```python
from build123d import *

# Parameters (mm, degrees)
SKETCH1_W                      = 155
SKETCH1_H                      = 290
BASE_FLANGE1_DEPTH             = 5
EDGE_FLANGE1_STRIP_W           = 36
EDGE_FLANGE1_STRIP_H           = 5
EDGE_FLANGE1_STRIP_CUT_DEPTH   = 290
EDGE_FLANGE1_STRIP_2_W         = 36
EDGE_FLANGE1_STRIP_2_H         = 5
EDGE_FLANGE1_STRIP_CUT_2_DEPTH = 290
EDGE_FLANGE1_DEPTH             = 290
EDGE_FLANGE1_BEND_DEPTH        = 290


# Sheet-metal steps are written as plain solids
with BuildPart() as part:
    # Sketch1 → Base-Flange1 (new body)
    with BuildSketch(Plane(origin=(0, 0, 0), x_dir=(1, 0, 0), z_dir=(0, 1, 0))):
        Rectangle(SKETCH1_W, SKETCH1_H)
    extrude(amount=-BASE_FLANGE1_DEPTH)

    # Edge-Flange1 strip (across the edge) → Edge-Flange1 strip cut (cut)
    with BuildSketch(Plane(origin=(77.5, -5, -145), x_dir=(-1, 0, 0), z_dir=(0, 0, 1))):
        with Locations((-5, -2.5)):
            Rectangle(EDGE_FLANGE1_STRIP_W, EDGE_FLANGE1_STRIP_H)
    extrude(amount=EDGE_FLANGE1_STRIP_CUT_DEPTH, mode=Mode.SUBTRACT)

    # Edge-Flange1 strip 2 (across the edge) → Edge-Flange1 strip cut 2 (cut)
    with BuildSketch(Plane(origin=(-77.5, -5, 145), x_dir=(1, 0, 0), z_dir=(0, 0, -1))):
        with Locations((-5, -2.5)):
            Rectangle(EDGE_FLANGE1_STRIP_2_W, EDGE_FLANGE1_STRIP_2_H)
    extrude(amount=EDGE_FLANGE1_STRIP_CUT_2_DEPTH, mode=Mode.SUBTRACT)

    # Edge-Flange1 section (across the edge) → Edge-Flange1 (add)
    with BuildSketch(Plane(origin=(77.5, -5, -145), x_dir=(-1, 0, 0), z_dir=(0, 0, 1))):
        with BuildLine():
            Line((0, 8), (0, 108))
            Line((0, 108), (5, 108))
            Line((5, 108), (5, 8))
            ThreePointArc((5, 8), (7.343145751, 2.343145751), (13, 0))
            Line((13, 0), (13, -5))
            ThreePointArc((13, -5), (3.807611845, -1.192388155), (0, 8))
        make_face()
    extrude(amount=EDGE_FLANGE1_DEPTH)

    # Edge-Flange1 section 2 (across the edge) → Edge-Flange1 bend (add)
    with BuildSketch(Plane(origin=(-77.5, -5, 145), x_dir=(1, 0, 0), z_dir=(0, 0, -1))):
        with BuildLine():
            Line((0, 8), (0, 108))
            Line((0, 108), (5, 108))
            Line((5, 108), (5, 8))
            ThreePointArc((5, 8), (7.343145751, 2.343145751), (13, 0))
            Line((13, 0), (13, -5))
            ThreePointArc((13, -5), (3.807611845, -1.192388155), (0, 8))
        make_face()
    extrude(amount=EDGE_FLANGE1_BEND_DEPTH)


solid = part.part
```
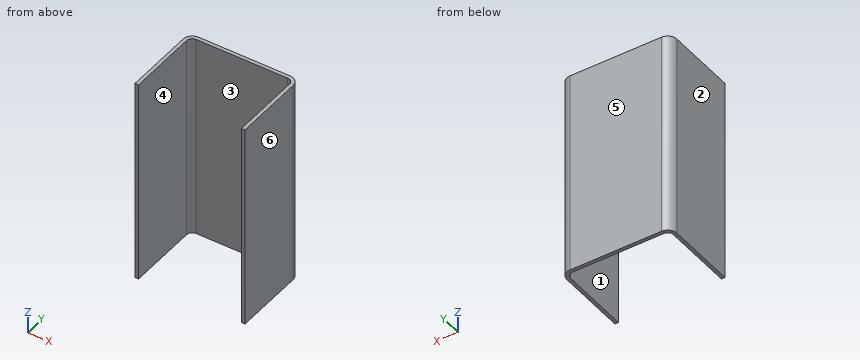
The model under review builds one solid part; all positions refer to its coordinate system, in mm. Face numbers are marked on the shaded views. A direction names the side the tool comes from. Round coordinates to 2 decimals unless told otherwise and drop trailing zeros. Order: outer loops, then holes, each group sorted by start corner. A loop starts at its lowest first (then second) coordinate and runs counter-clockwise, first axis right, second up. Notation, with made-up numbers: (-15, -6) - (39, -6) arc R35 ccw to (39, 29) - close; hole circle Ø11 at (83, 50). An arc over 180 degrees is marked (long way). Answer in a Markdown table with one row per item.
(1) Take a section at C-C on x = -28.5. Write out the cut boundary in (y, z), plus the area to 3 significant figures.
Result set:
| item | result |
|---|---|
| outline | (-5, -145) - (0, -145) - (0, 145) - (-5, 145) - close |
| area | 1,450 mm2 |
(2) Take a section at B-B on z = -91.5. Write out the cut boundary in (x, y).
Result set:
| item | result |
|---|---|
| outline | (-77.5, -113) - (-72.5, -113) - (-72.5, -13) arc R8 cw to (-64.5, -5) - (64.5, -5) arc R8 cw to (72.5, -13) - (72.5, -113) - (77.5, -113) - (77.5, -13) arc R13 ccw to (64.5, 0) - (-64.5, 0) arc R13 ccw to (-77.5, -13) - close |
(3) Clearance check with a flat-ended pin moving along its axis: P1, Ø6, axis at x = 9.5, z = -14.5, coming from the -Y side. State where the tip first meets the part, or that it passes through.
Result set:
| item | result |
|---|---|
| P1 | stops at y = -5 |
(4) Mouldability with a two-part tool opening along X and no side actions: class the marked faces 3, 4, 5 and 6 as released by +X, released by -X, zero draft, split by the parting line, or undercut.
Result set:
| item | result |
|---|---|
| face 3 | undercut |
| face 4 | undercut |
| face 5 | zero draft |
| face 6 | released by +X |
(5) Take a section at D-D on y = -9. Write out the cut boundary in (x, z), plus the area to 3 significant figures.
Result set:
| item | result |
|---|---|
| outline | (-76.87, -145) - (-71.43, -145) - (-71.43, 145) - (-76.87, 145) - close; (71.43, -145) - (76.87, -145) - (76.87, 145) - (71.43, 145) - close |
| area | 3,160 mm2 |
(6) Machinability: for the marked faces 1 and 2, which of the approach directions +Z, -Z, +X, -X, +Y, -Y give a long, thin tool a straight path to every point of the face, cutting with its end or side? Answer none if there is none.
Result set:
| item | result |
|---|---|
| face 1 | +Z, -Z, -Y |
| face 2 | +Z, -Z, -X, +Y, -Y |
(7) For line 1 (X direction, y = -26.5, z = -100); line 2 (Y direction, x = 8.5, z = 93); line 3 (Y direction, x = -68.5, z = -28), list the stretches that pass through material, from the lowest coordinate up. Write a range as from..to.
Result set:
| item | result |
|---|---|
| line 1 | x = -77.5..-72.5, 72.5..77.5 |
| line 2 | y = -5..0 |
| line 3 | y = -6.07..-0.63 |
(8) Take a section at A-A on y = -55. Write out the cut boundary in (x, z).
Result set:
| item | result |
|---|---|
| outline | (-77.5, -145) - (-72.5, -145) - (-72.5, 145) - (-77.5, 145) - close; (72.5, -145) - (77.5, -145) - (77.5, 145) - (72.5, 145) - close |
